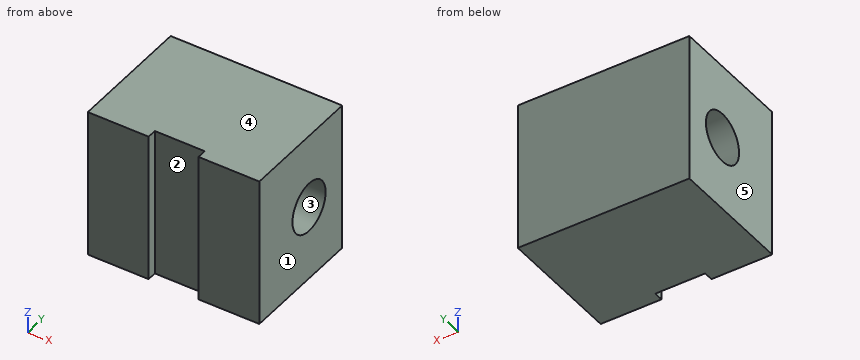
from build123d import *

# Parameters (mm, degrees)
SKETCH1_W           = 87.3125
SKETCH1_H           = 76.2
BOSS_EXTRUDE1_DEPTH = 63.5
SKETCH2_W           = 25.4
SKETCH2_H           = 76.2
CUT_EXTRUDE1_DEPTH  = 4.7625
SKETCH3_R           = 12.7
CUT_EXTRUDE2_DEPTH  = 88.3125


with BuildPart() as part:
    # Sketch1 → Boss-Extrude1 (new body)
    with BuildSketch(Plane(origin=(0, 0, 0), x_dir=(1, 0, 0), z_dir=(0, 1, 0))):
        Rectangle(SKETCH1_W, SKETCH1_H)
    extrude(amount=BOSS_EXTRUDE1_DEPTH)

    # Sketch2 → Cut-Extrude1 (cut)
    with BuildSketch(Plane.XZ):
        Rectangle(SKETCH2_W, SKETCH2_H)
    extrude(amount=-CUT_EXTRUDE1_DEPTH, mode=Mode.SUBTRACT)

    # Sketch3 → Cut-Extrude2 (cut, through all)
    with BuildSketch(Plane(origin=(43.65625, 0, 0), x_dir=(0, 0, -1), z_dir=(1, 0, 0))):
        with Locations((0, 38.1)):
            Circle(SKETCH3_R)
    extrude(amount=-CUT_EXTRUDE2_DEPTH, mode=Mode.SUBTRACT)


solid = part.part
For this review, take the finished solid that the model builds, in its own axes (mm). Face numbers are marked on the shaded views. A direction names the side the tool comes from. Round coordinates to 2 decimals unless told otherwise and drop trailing zeros. Loops run counter-clockwise (first coordinate to the right, second up) from the corner with the lowest first, then second, coordinate; pieces in that order, holes last. Notation, with made-up numbers: (22.25, 3.25) - (49.25, 3.25) arc R17 ccw to (49.25, 20.25) - close; hole circle Ø10 at (23, 19). An arc over 180 degrees is marked (long way). Put each result on its own line as item: value. Start each with the question number.
1. Mouldability with a two-part tool opening along Z and no side actions: class the marked faces 3, 4 and 5 as +Z half, -Z half, draft (parallel to the pull), parting line (faces both ways), or undercut.
2. Consider section C-C on x = 3. State the section outline as (y, z) points.
3. Insertion check: P1, Ø12, axis at x = -13.5, z = -11, coming from the -Y side. The pin has a flat end and moves straight along its axis. Give the tip position at first contact, or say it passes through.
4. Consider section B-B on y = 38.1. State the section outline as (x, z) points, plus the area to 3 significant figures.
5. Consider section A-A on z = 0. State the section outline as (x, y) points, plus the area to 3 significant figures.
6. For the marked faces 1 and 2, list the 3-axis set-ups (+Z, -Z, +X, -X, +Y, -Y) from which the entire face can be reached by the end or side of a thin tool; tool diameter is ignored.
7. For probe 1 along Z at (x, y) = (0, 38); probe 2 along Y at (x, z) = (18, 0); probe 3 along Y at (x, z) = (-30, 5), list the stretches that pass through material, from the lowest coordinate up. Write a range as [from, to].
8. Consider section D-D on z = 15.5. State the section outline as (x, y) points.
Result sheet:
1. face 3: undercut
1. face 4: +Z half
1. face 5: draft
2. outline: (4.76, -38.1) - (63.5, -38.1) - (63.5, 38.1) - (4.76, 38.1) - close; hole circle Ø25.4 at (38.1, 0)
3. P1: y = 0
4. outline: (-43.66, -38.1) - (43.66, -38.1) - (43.66, -12.7) - (-43.66, -12.7) - close; (-43.66, 12.7) - (43.66, 12.7) - (43.66, 38.1) - (-43.66, 38.1) - close
4. area: 4,440 mm^2
5. outline: (-43.66, 0) - (-12.7, 0) - (-12.7, 4.76) - (12.7, 4.76) - (12.7, 0) - (43.66, 0) - (43.66, 25.4) - (-43.66, 25.4) - close; (-43.66, 50.8) - (43.66, 50.8) - (43.66, 63.5) - (-43.66, 63.5) - close
5. area: 3,210 mm^2
6. face 1: +Z, -Z, +X, +Y, -Y
6. face 2: +Z, -Z, -Y
7. probe 1: [-38.1, -12.7], [12.7, 38.1]
7. probe 2: [0, 25.4], [50.8, 63.5]
7. probe 3: [0, 26.43], [49.77, 63.5]
8. outline: (-43.66, 0) - (-12.7, 0) - (-12.7, 4.76) - (12.7, 4.76) - (12.7, 0) - (43.66, 0) - (43.66, 63.5) - (-43.66, 63.5) - close
